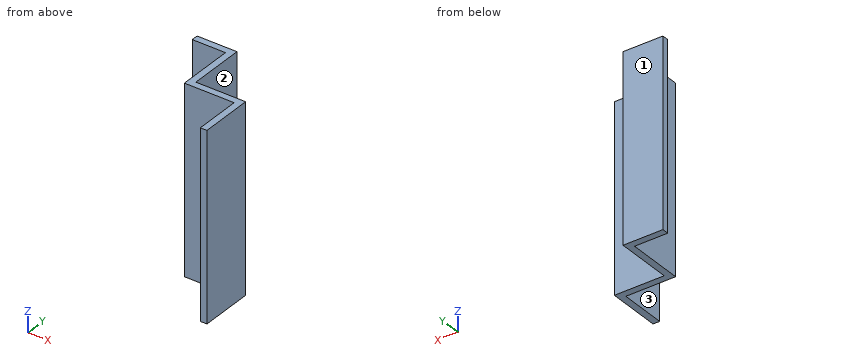
```python
from build123d import *

# Parameters (mm, degrees)
F0_W     = 38.1
F0_H     = 177.8
F1_DEPTH = 6.35
F2_W     = 6.35
F2_H     = 177.8
F3_DEPTH = 53.975
F4_W     = 6.35
F4_H     = 177.8
F5_DEPTH = 47.625
F6_W     = 6.35
F6_H     = 177.8
F7_DEPTH = 44.45


with BuildPart() as f1:
    # F0 (on Front) → F1 (new body)
    with BuildSketch(Plane.XZ):
        with Locations((-19.05, -88.9)):
            Rectangle(F0_W, F0_H)
    extrude(amount=F1_DEPTH)

    # F2 (on face) → F3 (join)
    with BuildSketch(Plane.XZ.offset(6.35)):
        with Locations((-3.175, -88.9)):
            Rectangle(F2_W, F2_H)
    extrude(amount=F3_DEPTH)

    # F4 (on face) → F5 (join)
    with BuildSketch(Plane.YZ):
        with Locations((-57.15, -88.9)):
            Rectangle(F4_W, F4_H)
    extrude(amount=F5_DEPTH)

    # F6 (on face) → F7 (join)
    with BuildSketch(Plane.XZ.offset(60.325)):
        with Locations((44.45, -88.9)):
            Rectangle(F6_W, F6_H)
    extrude(amount=F7_DEPTH)


solid = f1.part
```
Model file for the job. Use its own axes, mm. Face numbers are marked on the shaded views. A direction names the side the tool comes from. Coordinates: 2 decimals unless noted, no trailing zeros. Loops run counter-clockwise (first coordinate to the right, second up) from the corner with the lowest first, then second, coordinate; pieces in that order, holes last. Notation, with made-up numbers: (33, 61) - (51, 61) arc R19 cw to (51, 86) - close; hole circle Ø4 at (15, 78). An arc over 180 degrees is marked (long way). Answer as a JSON object with one key per item and string values. Group by question number.
(1) Tool access for the marked faces 1, 2 and 3: list every direction of +Z, -Z, +X, -X, +Y, -Y with a clear straight run to the whole face (end or side of a thin tool).
(2) Cut at A-A (z = -53). Give the cut face in (x, y) (3 decimals).
(3) Cut at B-B (y = -58.5). Give the cut face in (x, z) (3 decimals).
(4) Probe line 1 along X through (y, z) = (-30, -104); line 2 along X through (y, z) = (-60, -88) (3 decimals). List the from-to ranges inside material, lowest first.
(5) Flat gauge pins, fed straight in: pin 1 (2 mm diameter, centred on x = 16, z = -118, fed in from +Y) (3 decimals); pin 2 (8 mm diameter, centred on x = -9.5, z = -155.5, fed in from -Y) (3 decimals); pin 3 (9.5 mm diameter, centred on x = -28, z = -114, fed in from -Y); pin 4 (1.5 mm diameter, centred on x = 26.5, y = -63, fed in from -Z). Where does each tip first touch, or does it go through?
(6) Cut at C-C (x = 32.5). Give the cut face in (y, z) (3 decimals).
Geometry says:
{
 "1": {"face 1": "+Z, -Z, +X, -X, +Y", "face 2": "+Z, -Z, +X, +Y", "face 3": "+Z, -Z, -X, -Y"},
 "2": {"outline": "(-38.1, -6.35) - (-6.35, -6.35) - (-6.35, -60.325) - (41.275, -60.325) - (41.275, -104.775) - (47.625, -104.775) - (47.625, -53.975) - (0, -53.975) - (0, 0) - (-38.1, 0) - close"},
 "3": {"outline": "(-6.35, -177.8) - (47.625, -177.8) - (47.625, 0) - (-6.35, 0) - close"},
 "4": {"line 1": "x = -6.35 to 0", "line 2": "x = -6.35 to 47.625"},
 "5": {"pin 1": "stops at y = -53.975", "pin 2": "stops at y = -60.325", "pin 3": "stops at y = -6.35", "pin 4": "passes through"},
 "6": {"outline": "(-60.325, -177.8) - (-53.975, -177.8) - (-53.975, 0) - (-60.325, 0) - close"}
}
